Can you work these out from the model? Positions are in its coordinate system, mm. A direction names the side the tool comes from. Round coordinates to 2 decimals unless told otherwise and drop trailing zeros. Order: outer loops, then holes, each group sorted by start corner. A loop starts at its lowest first (then second) coordinate and runs counter-clockwise, first axis right, second up. Notation, with made-up numbers: (-24.75, 59) - (6.25, 59) arc R32 ccw to (6.25, 94) - close; hole circle Ø5 at (-2, 25). An arc over 180 degrees is marked (long way). Write item = value, one per line.
from build123d import *

# Parameters (mm, degrees)
AUFSATZ_LINEAR_AUSTRAGEN1_DEPTH = 40
SKIZZE2_W                       = 38
SKIZZE2_H                       = 15
SKIZZE2_R                       = 2
AUFSATZ_LINEAR_AUSTRAGEN2_DEPTH = 5


with BuildPart() as part:
    # Skizze1 → Aufsatz-Linear austragen1 (new body)
    with BuildSketch(Plane.XY):
        Polygon((-16, 1.942512926), (-13, 1.942512926), (-13, -2.057487074), (-14.916666667, -2.057487074), (-14.916666667, -5.057487074), (14.916666667, -5.057487074), (14.916666667, -2.057487074), (13, -2.057487074), (13, 1.942512926), (16, 1.942512926), (16, 3.609179593), (19, 3.609179593), (19, -9.057487074), (-19, -9.057487074), (-19, 3.609179593), (-16, 3.609179593), align=None)
    extrude(amount=AUFSATZ_LINEAR_AUSTRAGEN1_DEPTH)

    # Skizze2 → Aufsatz-Linear austragen2 (add)
    with BuildSketch(Plane(origin=(0, 0, 0), x_dir=(-1, 0, 0), z_dir=(0, 0, -1))):
        with Locations((0, -1.557487074)):
            Rectangle(SKIZZE2_W, SKIZZE2_H)
        Circle(SKIZZE2_R, mode=Mode.SUBTRACT)
    extrude(amount=AUFSATZ_LINEAR_AUSTRAGEN2_DEPTH)


solid = part.part
(1) If we section it at B-B (y = 0): Write out the boundary of the cut face in (x, z).
Computed:
outline = (-19, -5) - (-2, -5) - (-2, 0) - (-13, 0) - (-13, 40) - (-19, 40) - close; (2, -5) - (19, -5) - (19, 40) - (13, 40) - (13, 0) - (2, 0) - close
(2) If we section it at C-C (z = 34): Write out the boundary of the cut face in (x, y).
Computed:
outline = (-19, -9.06) - (19, -9.06) - (19, 3.61) - (16, 3.61) - (16, 1.94) - (13, 1.94) - (13, -2.06) - (14.92, -2.06) - (14.92, -5.06) - (-14.92, -5.06) - (-14.92, -2.06) - (-13, -2.06) - (-13, 1.94) - (-16, 1.94) - (-16, 3.61) - (-19, 3.61) - close
(3) On a 3-axis mill with a long thin cutter (end or side, diameter ignored), from which of +Z, -Z, +X, -X, +Y, -Y can I reach the whole of each face in a straight line? I mean faces 1 (the face through (0.3, -5.5, 40)), 2 (the face through (-14.917, -4, 20)), 3 (the face through (-16, 3, 20)), 4 (the face through (17, 3.609, 20)). Say none if no direction works.
Computed:
face_1 = +Z, +X, -X, +Y, -Y
face_2 = +Z
face_3 = +Z, +Y
face_4 = +Z, +X, -X, +Y
(4) If we section it at D-D (y = -3.25): Write out the boundary of the cut face in (x, z).
Computed:
outline = (-19, -5) - (19, -5) - (19, 40) - (14.92, 40) - (14.92, 0) - (-14.92, 0) - (-14.92, 40) - (-19, 40) - close
(5) Will these pins go through, and if not, where does the flat tip stop? P1, Ø3.5, axis at x = -14.5, z = 13.5, coming from the +Y side; P2, Ø5, axis at x = 1, y = 1, coming from the +Z side; P3, Ø1, axis at x = 4.5, z = 35.5, coming from the +Y side.
Computed:
P1 = 3.61
P2 = 0
P3 = -5.06
(6) If I drill on line 1 (Y direction, x = 0, z = -3); line 2 (X direction, y = -2.5, z = 7.5); line 3 (Y direction, x = 1.5, z = 19.5), over which ranges is the centre line in solid material (lowest first)? Write a range as from..to.
Computed:
line_1 = -9.06..-2, 2..5.94
line_2 = -19..-14.92, 14.92..19
line_3 = -9.06..-5.06
(7) If we section it at A-A (x = 0): Write out the boundary of the cut face in (y, z), plus the area to 3 significant figures.
Computed:
outline = (-9.06, -5) - (-2, -5) - (-2, 0) - (-5.06, 0) - (-5.06, 40) - (-9.06, 40) - close; (2, -5) - (5.94, -5) - (5.94, 0) - (2, 0) - close
area = 215 mm^2
